For this review, take the finished solid that the model builds, in its own axes (mm). Face numbers are marked on the shaded views. Round coordinates to 2 decimals unless told otherwise and drop trailing zeros. Write each loop counter-clockwise with the first axis right and the second up, starting at its lowest first coordinate (ties: lowest second). Pieces come first, ordered by that corner, then holes. Notation, with made-up numbers: M -10.75,-12.75 L 38.25,-12.75 A32 ccw 38.25,26.25 Z; hole C 31.25,66.5 d5. An arc over 180 degrees is marked long. Answer in a Markdown table with one row per item.
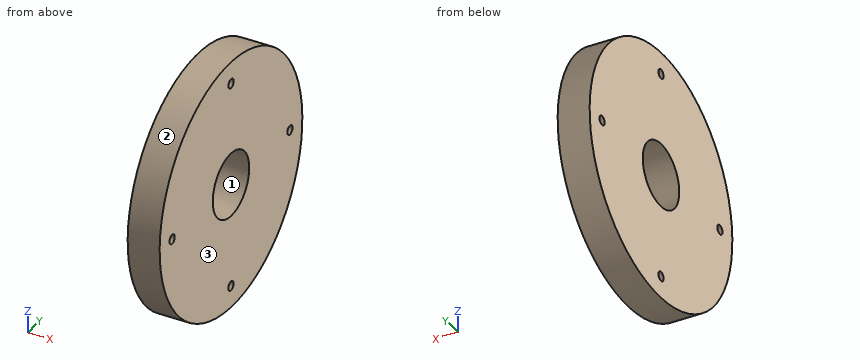
```python
from build123d import *

# Parameters (mm, degrees)
BOSS_EXTRUDE1_DEPTH      = 3.175
BOSS_EXTRUDE1_DEPTH_BACK = 3.175
SKETCH1_R                = 24.892
SKETCH1_R_2              = 6.3627
SKETCH2_R                = 0.916354932
CUT_EXTRUDE1_DEPTH       = 36.77073983
CIRPATTERN1_COUNT        = 4


with BuildPart() as part:
    # Sketch1 → Boss-Extrude1 (new, two sides: drawn at the far end of the back side and taken through both)
    with BuildSketch(Plane(origin=(0, 0, 0), x_dir=(0, 0, -1), z_dir=(1, 0, 0)).offset(-BOSS_EXTRUDE1_DEPTH_BACK)):
        Circle(SKETCH1_R)
        Circle(SKETCH1_R_2, mode=Mode.SUBTRACT)
    extrude(amount=BOSS_EXTRUDE1_DEPTH + BOSS_EXTRUDE1_DEPTH_BACK)

    # Sketch2 → Cut-Extrude1 (cut, symmetric)
    with BuildSketch(Plane(origin=(3.175, 0, 0), x_dir=(0, 0, -1), z_dir=(1, 0, 0))):
        with Locations((0, 20.546808672)):
            Circle(SKETCH2_R)
    cut_extrude1 = extrude(amount=CUT_EXTRUDE1_DEPTH, both=True, mode=Mode.SUBTRACT)

    # CirPattern1: Cut-Extrude1 ×4 about axis
    cirpattern1_axis = Axis((0, 0, 0), (1, 0, 0))
    for i in range(1, CIRPATTERN1_COUNT):
        add(cut_extrude1.rotate(cirpattern1_axis, i * 360 / CIRPATTERN1_COUNT), mode=Mode.SUBTRACT)


solid = part.part
```
Q1. Take a section at A-A (y = 0). State the section outline as (x, z) points (3 decimals), then the cut area to 3 significant figures.
Found:
| item | result |
|---|---|
| outline | M -3.175,-24.892 L 3.175,-24.892 L 3.175,-21.463 L -3.175,-21.463 Z; M -3.175,-19.63 L 3.175,-19.63 L 3.175,-6.363 L -3.175,-6.363 Z; M -3.175,6.363 L 3.175,6.363 L 3.175,19.63 L -3.175,19.63 Z; M -3.175,21.463 L 3.175,21.463 L 3.175,24.892 L -3.175,24.892 Z |
| area | 212 mm² |
Q2. Insertion check: P1, Ø1.6, axis at y = -20.55, z = 0, coming from the -X side; P2, Ø2, axis at x = 1, z = -8.5, coming from the -Y side. Each pin has a flat end and moves straight along its axis. Give the tip position at first contact, or say it passes through.
Found:
| item | result |
|---|---|
| P1 | through |
| P2 | y = -23.74 |
Q3. For probe 1 along Y at (x, z) = (-2.5, 0); probe 2 along Y at (x, z) = (-1.25, 0.5); probe 3 along Y at (x, z) = (-0.75, 2), list the stretches that pass through material, from the lowest coordinate up.
Found:
| item | result |
|---|---|
| probe 1 | -24.89 to -21.46, -19.63 to -6.36, 6.36 to 19.63, 21.46 to 24.89 |
| probe 2 | -24.89 to -21.31, -19.78 to -6.34, 6.34 to 19.78, 21.31 to 24.89 |
| probe 3 | -24.81 to -6.04, 6.04 to 24.81 |
Q4. Take a section at D-D (x = 1). State the section outline as (y, z) points.
Found:
| item | result |
|---|---|
| outline | C 0,0 d49.78; hole C -20.55,0 d1.83; hole C 0,0 d12.73; hole C 0,-20.55 d1.83; hole C 0,20.55 d1.83; hole C 20.55,0 d1.83 |
Q5. Take a section at C-C (z = -5.5). State the section outline as (x, y) points (3 decimals).
Found:
| item | result |
|---|---|
| outline | M -3.175,-24.277 L 3.175,-24.277 L 3.175,-3.199 L -3.175,-3.199 Z; M -3.175,3.199 L 3.175,3.199 L 3.175,24.277 L -3.175,24.277 Z |
Q6. Mouldability with a two-part tool opening along Y and no side actions: class the marked faces 1, 2 and 3 as +Y half, -Y half, draft (parallel to the pull), parting line (faces both ways), or undercut.
Found:
| item | result |
|---|---|
| face 1 | undercut |
| face 2 | parting line |
| face 3 | draft |
